from build123d import *

# Parameters (mm, degrees)
ESQUISSE1_W             = 12.5
ESQUISSE1_H             = 70
BOSS_EXTRU_1_DEPTH      = 10
ESQUISSE2_W             = 12.5
ESQUISSE2_H             = 12.576917286
BOSS_EXTRU_2_DEPTH      = 35
ENL_V_MAT_EXTRU_1_DEPTH = 40
CONG_1_R                = 10
CONG_3_R                = 2
D_GAGEMENT_M71_D        = 7.6
D_GAGEMENT_M71_DEPTH    = 12.5
D_GAGEMENT_M71_TIP      = 2.283270352


with BuildPart() as part:
    # Esquisse1 → Boss.-Extru.1 (new body)
    with BuildSketch(Plane.XY):
        Rectangle(ESQUISSE1_W, ESQUISSE1_H)
    extrude(amount=BOSS_EXTRU_1_DEPTH)

    # Esquisse2 → Boss.-Extru.2 (add)
    with BuildSketch(Plane(origin=(0, 0, 0), x_dir=(-1, 0, 0), z_dir=(0, 0, -1))):
        Rectangle(ESQUISSE2_W, ESQUISSE2_H)
    extrude(amount=-BOSS_EXTRU_2_DEPTH)

    # Esquisse3 → Enlèv. mat.-Extru.1 (cut)
    with BuildSketch(Plane(origin=(0, 0, 0), x_dir=(-1, 0, 0), z_dir=(0, 0, -1))):
        Polygon((-3.889087297, 0), (0, 3.889087297), (3.889087297, 0), (0, -3.889087297), align=None)
    extrude(amount=-ENL_V_MAT_EXTRU_1_DEPTH, mode=Mode.SUBTRACT)

    # Congé1
    cong_1_edges = [part.edges().sort_by_distance(p)[0] for p in [
        (0, -6.288458643, 10),
        (0, 6.288458643, 10),
    ]]
    fillet(cong_1_edges, radius=CONG_1_R)

    # Congé3
    cong_3_edges = [part.edges().sort_by_distance(p)[0] for p in [
        (0, -35, 10),
        (0, -35, 0),
        (0, 35, 0),
        (0, 35, 10),
    ]]
    fillet(cong_3_edges, radius=CONG_3_R)

    # Dégagement M71
    with Locations(Plane.ZY.offset(6.25)):
        with Locations((8.344762473, 0)):
            Hole(D_GAGEMENT_M71_D / 2, depth=D_GAGEMENT_M71_DEPTH)
            with Locations((0, 0, -(D_GAGEMENT_M71_DEPTH + D_GAGEMENT_M71_TIP / 2))):  # 118° drill point
                Cone(0, D_GAGEMENT_M71_D / 2, D_GAGEMENT_M71_TIP, mode=Mode.SUBTRACT)


solid = part.part
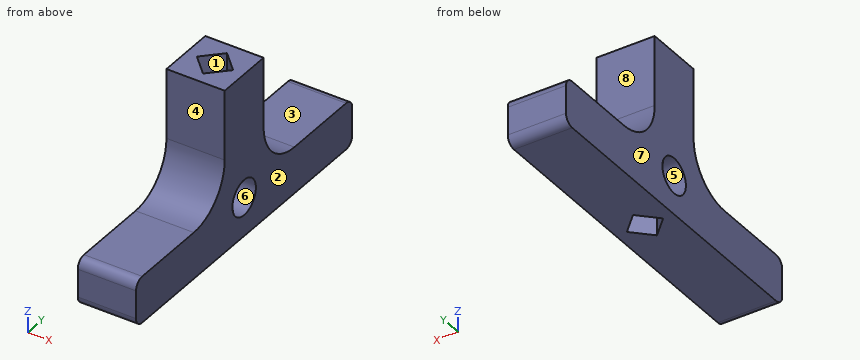
Source: CAD feature listing. Evaluate the final solid. Frame: model axes, mm. Face numbers are marked on the shaded views. A direction names the side the tool comes from. Give positions to 0.01 mm unless a question says otherwise; leave off trailing zeros. Write each loop counter-clockwise with the first axis right and the second up, starting at its lowest first coordinate (ties: lowest second). Pieces come first, ordered by that corner, then holes. Notation, with made-up numbers: M 36,65 L 47,65 A12 ccw 47,77 Z; hole C 52.25,49.5 d4. An arc over 180 degrees is marked long. Answer as a JSON object with one key per item and string values.
Q1. Ray query, line 1 along Y through (x, z) = (4.5, 8); line 2 along Z through (x, y) = (-4.5, 0); line 3 along Y through (x, z) = (-5.25, 26.5). Return the intervals inside material, ascending.
Geometry check:
{"line 1": "y = -35 to -3.78, 3.78 to 35", "line 2": "z = 0 to 4.54, 12.14 to 35", "line 3": "y = -6.29 to 6.29"}
Q2. Cut plane C-C, the plane z = 9. Return the cut outline in (x, y), then the cut area to 3 significant figures.
Geometry check:
{"outline": "M -6.25,-34.73 L 6.25,-34.73 L 6.25,-3.74 L 0.15,-3.74 L 0,-3.89 L -0.15,-3.74 L -6.25,-3.74 Z; M -6.25,3.74 L -0.15,3.74 L 0,3.89 L 0.15,3.74 L 6.25,3.74 L 6.25,34.73 L -6.25,34.73 Z", "area": "775 mm^2"}
Q3. Cut plane B-B, the plane y = -2.5. Return the cut outline in (x, z), then the cut area to 3 significant figures.
Geometry check:
{"outline": "M -6.25,0 L -1.39,0 L -1.39,5.48 L -6.25,5.48 Z; M -6.25,11.21 L -1.39,11.21 L -1.39,35 L -6.25,35 Z; M 1.39,0 L 6.25,0 L 6.25,5.48 L 1.39,5.48 Z; M 1.39,11.21 L 6.25,11.21 L 6.25,35 L 1.39,35 Z", "area": "285 mm^2"}
Q4. Cut plane D-D, the plane y = -20.5. Return the cut outline in (x, z), then the cut area to 3 significant figures.
Geometry check:
{"outline": "M -6.25,0 L 6.25,0 L 6.25,10 L -6.25,10 Z", "area": "125 mm^2"}
Q5. Contact query for flat-ended pins moving along their axis: P1, Ø3, axis at x = -2.5, z = 27.5, coming from the +Y side; P2, Ø3, axis at x = -2.5, z = 25, coming from the -Y side; P3, Ø6, axis at x = -1.5, y = 24, coming from the +Z side. Output: stop coordinate, or through.
Geometry check:
{"P1": "stops at y = 6.29", "P2": "stops at y = -6.29", "P3": "stops at z = 10"}
Q6. Access query for the marked faces 1, 2, 3, 4 and 5. Directions: +Z, -Z, +X, -X, +Y, -Y. A direction counts if a zero-diameter tool reaches every point of the face in a straight line with its end or side. Return the directions, or none.
Geometry check:
{"face 1": "+Z, -Z", "face 2": "+Z, -Z, +X, +Y, -Y", "face 3": "+Z, +X, -X, +Y", "face 4": "+Z, +X, -X, -Y", "face 5": "+X, -X"}
Q7. Cut plane A-A, the plane z = 22.5. Return the cut outline in (x, y).
Geometry check:
{"outline": "M -6.25,-6.29 L 6.25,-6.29 L 6.25,6.29 L -6.25,6.29 Z; hole M -3.89,0 L 0,-3.89 L 3.89,0 L 0,3.89 Z"}
Q8. Mould query, pull axis Y, two halves, no side actions, for the marked faces 6, 7 and 8. Classes: +Y half, -Y half, draft (parallel to the pull), parting line (faces both ways), or undercut.
Geometry check:
{"face 6": "undercut", "face 7": "draft", "face 8": "+Y half"}
